Geometry: final body of the model. Coordinates: model frame, mm. A direction names the side the tool comes from. Give positions to 0.01 mm unless a question says otherwise; leave off trailing zeros. Write each loop counter-clockwise with the first axis right and the second up, starting at its lowest first coordinate (ties: lowest second). Pieces come first, ordered by that corner, then holes. Notation, with made-up numbers: (66, -19.75) -> (78, -19.75) arc R30 ccw to (78, 14.25) -> close; hole circle Ø3 at (13, 35). An arc over 180 degrees is marked (long way). Use CSV: the item, a comma, the result in double quotes. Start each with the question number.
1) Material intervals for line 1 (X direction, y = -6.75, z = -22.5); line 2 (Z direction, x = 36, y = -5.75); line 3 (Z direction, x = 26.5, y = -5), sorted ascending. Write a range as [from, to].
2) Draft query along Z for faces 1 (the face through (0, -14, 0)), 2 (the face through (49.5, -13.5, 31.75)), 3 (the face through (9.01, -1.61, -21.56)), 4 (the face through (19.4, -16.95, 0.37)). Return one class per face: pulls with the +Z half, pulls with the -Z half, needs draft (parallel to the pull), parting line crosses it, or undercut.
3) Contact query for flat-ended pins moving along their axis: P1, Ø4, axis at x = 41, z = -2.5, coming from the +Y side; P2, Ø4, axis at x = 7.5, y = -1.5, coming from the +Z side; P3, Ø2.5, axis at y = -3.5, z = 19, coming from the +X side; P4, Ø12, axis at x = 25, z = 23, coming from the +Y side. Output: stop coordinate, or through.
4) Section C-C (y = -8). Output: boundary loops of the cut face in (x, z).
5) Set-up query: faces 5 (the face through (1, -5.08, -20)), 6 (the face through (15, -5.08, 20)), 7 (the face through (56.247, -16.056, 0.444)), 8 (the face through (6, -3.175, -20)), 9 (the face through (14.224, -4, 20)). Return all of +Z, -Z, +X, -X, +Y, -Y with unobstructed straight access to the full face (end or side cutting, diameter ignored); none if empty.
6) Section B-B (y = -1). Count the separate pieces of the cut face and the enclosed holes in it, plus the area to 3 significant figures.
7) Section D-D (x = 41). Output: boundary loops of the cut face in (y, z), plus the area to 3 significant figures.
8) Section A-A (z = -18). Output: boundary loops of the cut face in (x, y) (1 decimal).
```python
from build123d import *

# Parameters (mm, degrees)
SKETCH1_R                = 16.9545
BOSS_EXTRUDE1_DEPTH      = 50.8
SKETCH2_R                = 16.9545
BOSS_EXTRUDE2_DEPTH      = 31.75
SKETCH3_R                = 13.081
CUT_EXTRUDE1_DEPTH       = 50.8
SKETCH5_R                = 13.081
CUT_EXTRUDE2_DEPTH       = 63.5
CUT_EXTRUDE4_DEPTH       = 77.72150833
CUT_EXTRUDE4_DEPTH_BACK  = 77.72150833
SKETCH6_R                = 3.81
BOSS_EXTRUDE3_REACH      = 91.447
BOSS_EXTRUDE3_END_RADIUS = 16.9545
SKETCH8_W                = 15.875
SKETCH8_H                = 5.08
CUT_EXTRUDE5_REACH       = 91.447
CUT_EXTRUDE5_END_RADIUS  = 16.9545
SKETCH9_W                = 12.573
SKETCH9_H                = 1.905
SKETCH10_R               = 1.5875
CUT_EXTRUDE6_DEPTH       = 77.08291144


with BuildPart() as part:
    # Sketch1 → Boss-Extrude1 (new body)
    with BuildSketch(Plane(origin=(0, 0, 0), x_dir=(0, 0, -1), z_dir=(1, 0, 0))):
        Circle(SKETCH1_R)
    extrude(amount=BOSS_EXTRUDE1_DEPTH)

    # Sketch2 → Boss-Extrude2 (add, symmetric)
    with BuildSketch(Plane.XY):
        with Locations((50.8, 0)):
            Circle(SKETCH2_R)
    extrude(amount=BOSS_EXTRUDE2_DEPTH, both=True)

    # Sketch3 → Cut-Extrude1 (cut)
    with BuildSketch(Plane.ZY):
        Circle(SKETCH3_R)
    extrude(amount=-CUT_EXTRUDE1_DEPTH, mode=Mode.SUBTRACT)

    # Sketch5 → Cut-Extrude2 (cut)
    with BuildSketch(Plane(origin=(0, 0, -31.75), x_dir=(-1, 0, 0), z_dir=(0, 0, -1))):
        with Locations((-50.8, 0)):
            Circle(SKETCH5_R)
    extrude(amount=-CUT_EXTRUDE2_DEPTH, mode=Mode.SUBTRACT)

    # Sketch6 → Cut-Extrude4 (cut, two sides: drawn at the far end of the back side and taken through both)
    with BuildSketch(Plane(origin=(0, 0, 0), x_dir=(0, 0, -1), z_dir=(1, 0, 0)).offset(-CUT_EXTRUDE4_DEPTH_BACK)):
        with Locations(Location((0, 0, 0), (0, 0, 180))):
            Circle(SKETCH6_R)
    extrude(amount=CUT_EXTRUDE4_DEPTH + CUT_EXTRUDE4_DEPTH_BACK, mode=Mode.SUBTRACT)

    # SurfaceCut1
    split(bisect_by=Plane(origin=(0, 0, 0), x_dir=(1, 0, 0), z_dir=(0, 1, 0)), keep=Keep.BOTTOM)


with BuildPart() as body_2:
    # Boss-Extrude3: up to this cylinder (the profile starts outside it)
    boss_extrude3_end = Plane(origin=(7.9375, 0, 0), z_dir=(-1, 0, 0)) * Cylinder(BOSS_EXTRUDE3_END_RADIUS, 217.803, mode=Mode.PRIVATE)
    # Sketch8 → Boss-Extrude3 (new, up to the surface)
    with BuildSketch(Plane.XY.offset(24.13), mode=Mode.PRIVATE) as boss_extrude3_sk1:
        with Locations((7.9375, -2.54)):
            Rectangle(SKETCH8_W, SKETCH8_H)
    boss_extrude3_tool1 = extrude(boss_extrude3_sk1.sketch, amount=-BOSS_EXTRUDE3_REACH, mode=Mode.PRIVATE) - boss_extrude3_end
    add(boss_extrude3_tool1.solids().sort_by_distance((7.9375, -2.54, 24.13))[0])

    # Cut-Extrude5: up to this cylinder (the profile starts outside it)
    cut_extrude5_end = Plane(origin=(7.9375, 0, 0), z_dir=(-1, 0, 0)) * Cylinder(CUT_EXTRUDE5_END_RADIUS, 217.803, mode=Mode.PRIVATE)
    # Sketch9 → Cut-Extrude5 (cut, up to the surface)
    with BuildSketch(Plane.XY.offset(24.13), mode=Mode.PRIVATE) as cut_extrude5_sk1:
        with Locations((7.9375, -4.1275)):
            Rectangle(SKETCH9_W, SKETCH9_H)
    cut_extrude5_tool1 = extrude(cut_extrude5_sk1.sketch, amount=-CUT_EXTRUDE5_REACH, mode=Mode.PRIVATE) - cut_extrude5_end
    add(cut_extrude5_tool1.solids().sort_by_distance((7.9375, -4.1275, 24.13))[0], mode=Mode.SUBTRACT)


with BuildPart() as body_3:
    # Mirror1: mirrored copy
    add(body_2.part.mirror(Plane.XY))


with BuildPart() as part_1:
    add(part.part)

    # Intersect1: read off the stored shape, not the designer's step
    # Intersect1: union body 3, body 2
    add(body_3.part)
    add(body_2.part)

    # Sketch10 → Cut-Extrude6 (cut, through all)
    with BuildSketch(Plane.XZ.offset(3.175)):
        with Locations(Location((7.9375, 20.392281148, 0), (0, 0, 270))):
            Circle(SKETCH10_R)
    cut_extrude6 = extrude(amount=-CUT_EXTRUDE6_DEPTH, mode=Mode.SUBTRACT)

    # Mirror2: Cut-Extrude6 across plane
    add(cut_extrude6.mirror(Plane.XY), mode=Mode.SUBTRACT)


solid = part_1.part
```
Answers follow:
1,line 1,"x = [35.25, 39.6], [62, 66.35]"
1,line 2,"z = [-31.75, -11.75], [11.75, 31.75]"
1,line 3,"z = [-16.2, -12.09], [12.09, 16.2]"
2,face 1,"needs draft"
2,face 2,"pulls with the +Z half"
2,face 3,"undercut"
2,face 4,"parting line crosses it"
3,P1,"stops at y = -12.28"
3,P2,"stops at z = 24.13"
3,P3,"stops at x = 67.6"
3,P4,"passes through"
4,outline,"(0, -14.95) -> (35.85, -14.95) -> (35.85, -31.75) -> (40.45, -31.75) -> (40.45, -10.35) -> (0, -10.35) -> close; (0, 10.35) -> (40.45, 10.35) -> (40.45, 31.75) -> (35.85, 31.75) -> (35.85, 14.95) -> (0, 14.95) -> close; (61.15, -31.75) -> (65.75, -31.75) -> (65.75, 31.75) -> (61.15, 31.75) -> close"
5,face 5,"-Z, -X, -Y"
5,face 6,"+Z, -X, -Y"
5,face 7,"-Y"
5,face 8,"-Z, -Y"
5,face 9,"+Z, -Y"
6,separate pieces,"4"
6,enclosed holes,"2"
6,area,"839 mm^2"
7,outline,"(-13.84, -31.75) -> (-8.66, -31.75) -> (-8.66, -9.8) arc R13.08 cw to (-8.66, 9.8) -> (-8.66, 31.75) -> (-13.84, 31.75) -> (-13.84, 9.8) arc R16.95 ccw to (-13.84, -9.8) -> close"
7,area,"310 mm^2"
8,outline,"(0, -5.1) -> (1.7, -5.1) -> (1.7, -3.2) -> (14.2, -3.2) -> (14.2, -5.1) -> (15.9, -5.1) -> (15.9, 0) -> (0, 0) -> close; (33.8, 0) arc R17 ccw to (67.8, 0) -> (63.9, 0) arc R13.1 cw to (37.7, 0) -> close"
